```python
from build123d import *

# Parameters (mm, degrees)
SKETCH_1_R      = 1
EXTRUDE_1_DEPTH = 3


with BuildPart() as part:
    # 草图1 → 凸台-拉伸1 (new body)
    with BuildSketch(Plane.XY):
        with BuildLine():
            Line((-470.172785233, 43.756242), (-470.172785233, 77.756242))
            ThreePointArc((-470.172785233, 77.756242), (-474.672785233, 82.256242), (-479.172785233, 77.756242))
            Line((-479.172785233, 77.756242), (-479.172785233, 43.756242))
            ThreePointArc((-479.172785233, 43.756242), (-474.672785233, 39.256242), (-470.172785233, 43.756242))
        make_face()
        with Locations((-474.672785233, 66.756242)):
            Circle(SKETCH_1_R, mode=Mode.SUBTRACT)
        with Locations((-474.672785233, 54.756242)):
            Circle(SKETCH_1_R, mode=Mode.SUBTRACT)
        with BuildLine():
            Line((-472.873395696, 72.756242), (-472.873395696, 47.675550149))
            ThreePointArc((-472.873395696, 47.675550149), (-473.24087984, 46.901002738), (-474.07324308, 46.695723112))
            ThreePointArc((-474.07324308, 46.695723112), (-476.996427467, 41.858694433), (-471.672785233, 43.756242))
            Line((-471.672785233, 43.756242), (-471.672174771, 72.756229357))
            ThreePointArc((-471.672174771, 72.756229357), (-472.272778912, 73.356852463), (-472.873395696, 72.756242))
        make_face(mode=Mode.SUBTRACT)
        with BuildLine():
            Line((-476.470594729, 48.756242), (-476.694432062, 73.880013915))
            ThreePointArc((-476.694432062, 73.880013915), (-476.308150012, 74.678479143), (-475.439050119, 74.855752709))
            ThreePointArc((-475.439050119, 74.855752709), (-472.295939145, 79.586707151), (-477.672785233, 77.756242))
            Line((-477.672785233, 77.756242), (-477.672785233, 48.807558702))
            ThreePointArc((-477.672785233, 48.807558702), (-477.09846695, 48.154599371), (-476.470594729, 48.756242))
        make_face(mode=Mode.SUBTRACT)
    extrude(amount=EXTRUDE_1_DEPTH)


solid = part.part
```
Check sheet for the modelled part. Datum: model origin and axes. Units: mm. A direction names the side the tool comes from. Round coordinates to 2 decimals unless told otherwise and drop trailing zeros. Write each loop counter-clockwise with the first axis right and the second up, starting at its lowest first coordinate (ties: lowest second). Pieces come first, ordered by that corner, then holes. Notation, with made-up numbers: M 50,4.25 L 104,4.25 A14 cw 104,27.25 Z; hole C -33,54 d4. An arc over 180 degrees is marked long. Write item = value, one per line. Start each with the question number.
1. Section check B-B, the plane y = 75.5. Record the cut outline in (x, z).
2. Release check for a two-part mould opening along Y. For faces 1 (the cylindrical face through (-473.75, 66.37, 1.48)), 2 (the cylindrical face through (-474.574, 82.255, 1.479)), 3 (the cylindrical face through (-474.772, 39.257, 1.479)), 4 (the flat face through (-475, 61, 0)) record: pulls with the +Y half, pulls with the -Y half, needs draft (parallel to the pull), parting line crosses it, or undercut.
3. Scan lines: line 1 (X direction, y = 49, z = 2.05); line 2 (Y direction, x = -475.5, z = 1); line 3 (X direction, y = 70, z = 1.05). Record each from-to range of solid material in increasing order. Write a range as [from, to].
4. Section check C-C, the plane z = 0.8. Record the cut outline in (x, y), then the cut area to 3 significant figures.
5. Tool access check on faces 5 (the cylindrical face through (-473.23, 46.91, 1.48)), 6 (the flat face through (-470.173, 61, 1)). Record the directions out of +Z, -Z, +X, -X, +Y, -Y that give a thin tool (end or side, any length) a straight path to the whole face; none if there is none.
6. Section check A-A, the plane x = -475. Record the cut outline in (y, z).
7. Gauge pin test, flat end, axial feed: pin 1 (1.5 mm diameter, centred on x = -476.5, z = 2, fed in from +Y). Record the tip position at first contact, or that the pin passes through.
8. Section check D-D, the plane y = 49.5. Record the cut outline in (x, z), then the cut area to 3 significant figures.
Results found:
q1.outline = M -479.17,0 L -477.67,0 L -477.67,3 L -479.17,3 Z; M -472.7,0 L -470.17,0 L -470.17,3 L -472.7,3 Z
q2.face_1 = undercut
q2.face_2 = pulls with the +Y half
q2.face_3 = pulls with the -Y half
q2.face_4 = needs draft
q3.line_1 = [-479.17, -477.67], [-476.47, -472.87], [-471.67, -470.17]
q3.line_2 = [39.33, 40.87], [46.64, 54.19], [55.32, 66.19], [67.32, 74.87], [80.64, 82.18]
q3.line_3 = [-479.17, -477.67], [-476.66, -472.87], [-471.67, -470.17]
q4.outline = M -479.17,43.76 A4.5 ccw -470.17,43.76 L -470.17,77.76 A4.5 ccw -479.17,77.76 Z; hole M -477.67,48.81 A0.6 ccw long -476.47,48.76 L -476.69,73.88 A1 cw -475.44,74.86 A3 ccw long -477.67,77.76 Z; hole C -474.67,54.76 d2; hole C -474.67,66.76 d2; hole M -474.07,46.7 A3 ccw long -471.67,43.76 L -471.67,72.76 A0.6 ccw -472.87,72.76 L -472.87,47.68 A1 cw Z
q4.area = 242 mm^2
q5.face_5 = +Z, -Z
q5.face_6 = +Z, -Z, +X, +Y, -Y
q6.outline = M 39.27,0 L 40.77,0 L 40.77,3 L 39.27,3 Z; M 46.74,0 L 53.81,0 L 53.81,3 L 46.74,3 Z; M 55.7,0 L 65.81,0 L 65.81,3 L 55.7,3 Z; M 67.7,0 L 74.77,0 L 74.77,3 L 67.7,3 Z; M 80.74,0 L 82.24,0 L 82.24,3 L 80.74,3 Z
q7.pin_1 = 82.13
q8.outline = M -479.17,0 L -477.67,0 L -477.67,3 L -479.17,3 Z; M -476.48,0 L -472.87,0 L -472.87,3 L -476.48,3 Z; M -471.67,0 L -470.17,0 L -470.17,3 L -471.67,3 Z
q8.area = 19.8 mm^2
